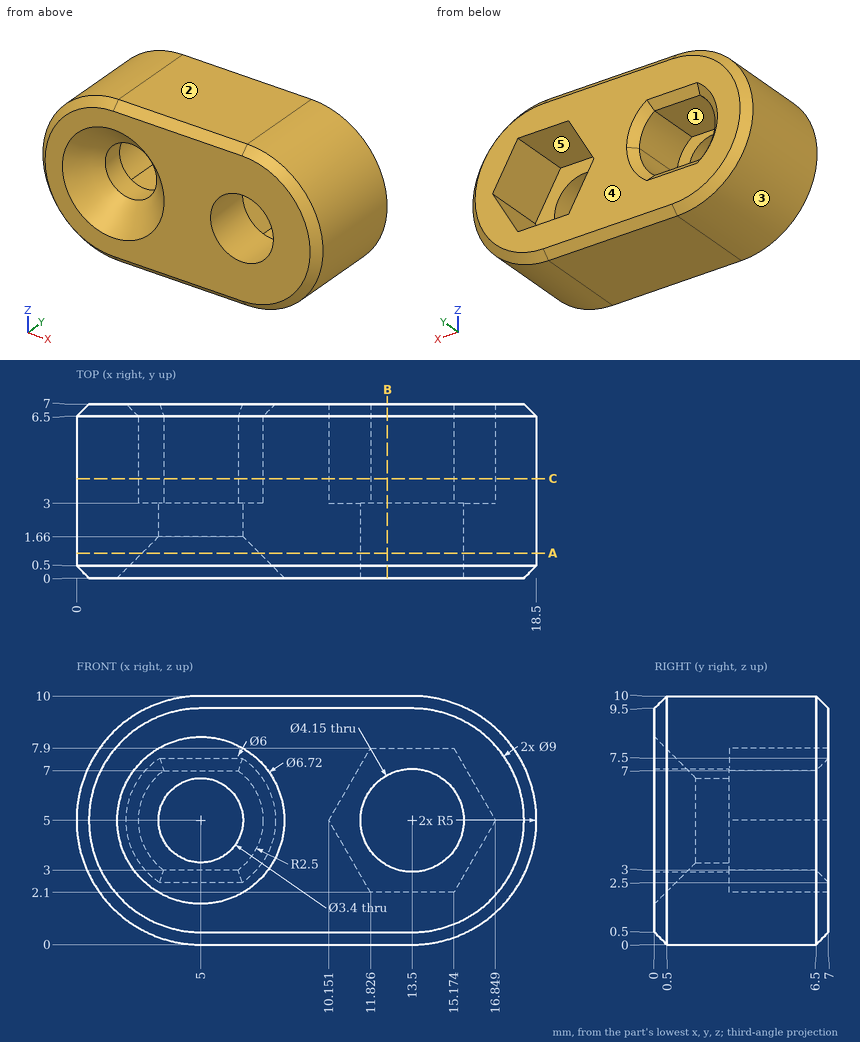
Source: three-view drawing plus pictorial views. Frame: mm from the lowest corner of the part. A direction names the side the tool comes from. Give positions to 0.01 mm unless a question says otherwise; leave off trailing zeros. Write each loop counter-clockwise with the first axis right and the second up, starting at its lowest first coordinate (ties: lowest second). Pieces come first, ordered by that corner, then holes. Notation, with made-up numbers: (23, 21) - (63, 21) arc R22 cw to (63, 30) - close; hole circle Ø11 at (49.5, 55). An arc over 180 degrees is marked (long way). Write item = value, one per line. Start each with the question number.
Q1. Cut plane C-C, the plane y = 4. Return loops of the section in (x, z) (1 decimal), then the cut area to 3 significant figures.
Q2. Draft query along X for the marked faces 1, 2 and 3. Return one class per face: +X half, -X half, draft (parallel to the pull), parting line (faces both ways), or undercut.
Q3. Reachability of the marked faces 4 and 5 from +Z, -Z, +X, -X, +Y, -Y: full face, straight path, thin tool, end or side. Return the list, or none.
Q4. Pin query (flat end, axial travel): pin 1 Ø1.7 at (x, z) = (14.5, 4) entering from +Y; pin 2 Ø3 at (x, z) = (4, 4.5) entering from +Y; pin 3 Ø5.5 at (x, z) = (5, 5) entering from -Y. Return the tip coordinate at first contact, or that it passes through.
Q5. Material intervals for probe 1 along X at (y, z) = (3.5, 6.25) (1 decimal); probe 2 along X at (y, z) = (1.25, 4.25) (1 decimal); probe 3 along Z at (x, y) = (5, 2.15), sorted ascending.
Q6. Cut plane B-B, the plane x = 12.5. Return loops of the section in (y, z).
Q7. Cut plane A-A, the plane y = 1. Give the number of separate pieces and of enclosed holes in the cut face.
Computed values:
q1.outline = (5, 0) - (13.5, 0) arc R5 ccw to (13.5, 10) - (5, 10) arc R5 ccw to start; hole (3.5, 3) - (6.5, 3) arc R2.5 ccw to (6.5, 7) - (3.5, 7) arc R2.5 ccw to start; hole (10.2, 5) - (11.8, 2.1) - (15.2, 2.1) - (16.8, 5) - (15.2, 7.9) - (11.8, 7.9) - close
q1.area = 117 mm²
q2.face_1 = undercut
q2.face_2 = draft
q2.face_3 = -X half
q3.face_4 = +Z, -Z, +X, -X, +Y
q3.face_5 = +Y
q4.pin_1 = 3
q4.pin_2 = 6.62
q4.pin_3 = 0.61
q5.probe_1 = 0.2 to 2.8, 7.2 to 10.9, 16.1 to 18.3
q5.probe_2 = 0.1 to 3, 7 to 11.6, 15.4 to 18.4
q5.probe_3 = 0 to 3.3, 6.7 to 10
q6.outline = (0, 0.5) - (0.5, 0) - (6.5, 0) - (7, 0.5) - (7, 2.1) - (3, 2.1) - (3, 3.18) - (0, 3.18) - close; (0, 6.82) - (3, 6.82) - (3, 7.9) - (7, 7.9) - (7, 9.5) - (6.5, 10) - (0.5, 10) - (0, 9.5) - close
q7.separate_pieces = 1
q7.enclosed_holes = 2
